```python
from build123d import *
from OCP.BRepFilletAPI import BRepFilletAPI_MakeChamfer

# Parameters (mm, degrees)
BOSS_EXTRUDE1_DEPTH = 3
CHAMFER1_SIZE       = 3
CHAMFER1_SIZE_2     = 1.853922924
SKETCH7_R           = 2
CUT_EXTRUDE6_DEPTH  = 1.5
SKETCH9_R           = 2
CUT_EXTRUDE7_DEPTH  = 1.5
SKETCH12_R          = 2
CUT_EXTRUDE8_DEPTH  = 1.5
SKETCH11_R          = 2
CUT_EXTRUDE9_DEPTH  = 1.5
SKETCH10_R          = 2
CUT_EXTRUDE10_DEPTH = 1.5


with BuildPart() as part:
    # Sketch1 → Boss-Extrude1 (new body)
    with BuildSketch(Plane(origin=(0, 0, 0), x_dir=(1, 0, 0), z_dir=(0, 1, 0))):
        Polygon((61.803398875, 0), (19.098300563, 58.778525229), (-50, 36.3271264), (-50, -36.3271264), (19.098300563, -58.778525229), align=None)
    extrude(amount=BOSS_EXTRUDE1_DEPTH)

    # Chamfer1
    chamfer1_edges_1 = [part.edges().sort_by_distance(p)[0] for p in [
        (-50, 3, 0),
    ]]
    chamfer1_side_1 = [part.faces().sort_by_distance(p)[0] for p in [
        (-50, 2.962921542, 0),
    ]]
    chamfer1_edges_2 = [part.edges().sort_by_distance(p)[0] for p in [
        (-15.450849719, 3, -47.552825815),
    ]]
    chamfer1_side_2 = [part.faces().sort_by_distance(p)[0] for p in [
        (-15.450849719, 2.962921542, -47.552825815),
    ]]
    chamfer1_edges_3 = [part.edges().sort_by_distance(p)[0] for p in [
        (40.450849719, 3, -29.389262615),
    ]]
    chamfer1_side_3 = [part.faces().sort_by_distance(p)[0] for p in [
        (40.450849719, 2.962921542, -29.389262615),
    ]]
    chamfer1_edges_4 = [part.edges().sort_by_distance(p)[0] for p in [
        (40.450849719, 3, 29.389262615),
    ]]
    chamfer1_side_4 = [part.faces().sort_by_distance(p)[0] for p in [
        (40.450849719, 2.962921542, 29.389262615),
    ]]
    chamfer1_edges_5 = [part.edges().sort_by_distance(p)[0] for p in [
        (-15.450849719, 3, 47.552825815),
    ]]
    chamfer1_side_5 = [part.faces().sort_by_distance(p)[0] for p in [
        (-15.450849719, 2.962921542, 47.552825815),
    ]]
    chamfer1 = BRepFilletAPI_MakeChamfer(part.part.solid().wrapped)
    for e in chamfer1_edges_1:
        chamfer1.Add(CHAMFER1_SIZE - 0.0001, CHAMFER1_SIZE_2 - 0.0001, e.wrapped, chamfer1_side_1[0].wrapped)
    for e in chamfer1_edges_2:
        chamfer1.Add(CHAMFER1_SIZE - 0.0001, CHAMFER1_SIZE_2 - 0.0001, e.wrapped, chamfer1_side_2[0].wrapped)
    for e in chamfer1_edges_3:
        chamfer1.Add(CHAMFER1_SIZE - 0.0001, CHAMFER1_SIZE_2 - 0.0001, e.wrapped, chamfer1_side_3[0].wrapped)
    for e in chamfer1_edges_4:
        chamfer1.Add(CHAMFER1_SIZE - 0.0001, CHAMFER1_SIZE_2 - 0.0001, e.wrapped, chamfer1_side_4[0].wrapped)
    for e in chamfer1_edges_5:
        chamfer1.Add(CHAMFER1_SIZE - 0.0001, CHAMFER1_SIZE_2 - 0.0001, e.wrapped, chamfer1_side_5[0].wrapped)
    add(Compound.cast(chamfer1.Shape()), mode=Mode.REPLACE)  # a hair under: the kernel refuses the full size

    # Sketch7 → Cut-Extrude6 (cut, along a direction that is not the sketch's normal)
    with BuildSketch(Plane.XZ):
        with Locations((16.806504495, -51.725102202)):
            Circle(SKETCH7_R)
    extrude(amount=-CUT_EXTRUDE6_DEPTH, dir=(0.18758103429764753, -0.7946827516361076, -0.5773150611441635), mode=Mode.SUBTRACT)

    # Sketch9 → Cut-Extrude7 (cut, along a direction that is not the sketch's normal)
    with BuildSketch(Plane.XZ):
        with Locations((-44, -31.967871232)):
            Circle(SKETCH9_R)
    extrude(amount=-CUT_EXTRUDE7_DEPTH, dir=(-0.4910935234360889, -0.7946827516361092, -0.356800330004317), mode=Mode.SUBTRACT)

    # Sketch12 → Cut-Extrude8 (cut, along a direction that is not the sketch's normal)
    with BuildSketch(Plane.XZ):
        with Locations((-44, 31.967871232)):
            Circle(SKETCH12_R)
    extrude(amount=-CUT_EXTRUDE8_DEPTH, dir=(-0.4910935234360893, -0.7946827516361098, 0.35680033000431516), mode=Mode.SUBTRACT)

    # Sketch11 → Cut-Extrude9 (cut, along a direction that is not the sketch's normal)
    with BuildSketch(Plane.XZ):
        with Locations((16.806504495, 51.725102202)):
            Circle(SKETCH11_R)
    extrude(amount=-CUT_EXTRUDE9_DEPTH, dir=(0.18758103429764547, -0.7946827516361094, 0.577315061144162), mode=Mode.SUBTRACT)

    # Sketch10 → Cut-Extrude10 (cut, along a direction that is not the sketch's normal)
    with BuildSketch(Plane.XZ):
        with Locations((54.38699101, 0)):
            Circle(SKETCH10_R)
    extrude(amount=-CUT_EXTRUDE10_DEPTH, dir=(0.607024978276895, -0.7946827516361074, -2.948455894095108e-15), mode=Mode.SUBTRACT)


solid = part.part
```
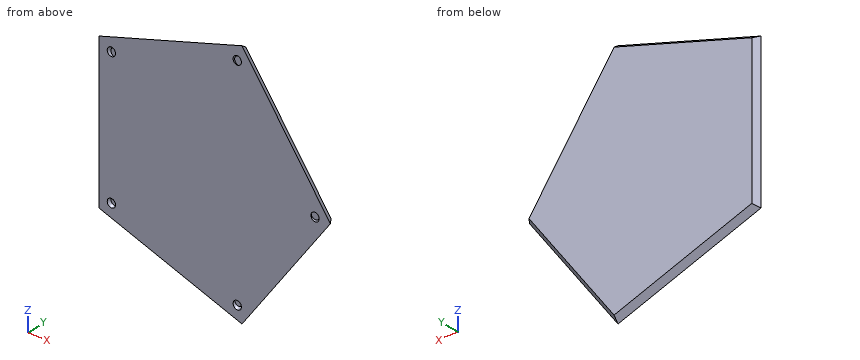
Here's how the part is built. I have some questions about the finished solid (model axes, mm). Coordinates: 2 decimals unless noted, no trailing zeros. Order: outer loops, then holes, each group sorted by start corner. A loop starts at its lowest first (then second) coordinate and runs counter-clockwise, first axis right, second up.
1) Will these pins go through, and if not, where does the flat tip stop? pin 1 (1.2 mm diameter, centred on x = 17, z = 50, fed in from -Y); pin 2 (1 mm diameter, centred on x = 2, y = 0.5, fed in from -Z); pin 3 (1.2 mm diameter, centred on x = -44, z = -32, fed in from -Y); pin 4 (1 mm diameter, centred on y = 1.5, z = -13, fed in from -X).
2) I need wall thicknesses on line 1 (Z direction, x = -43.5, y = 0.95); line 2 (Z direction, x = 40, y = 1.25); line 3 (Z direction, x = 42.5, y = 2.25). Which ranges of each line are inside material? Lowest first, please.
3) Imagine slicing it at A-A on y = 1.75. List the corners of the cut face in (x, z) for me, and give its area (3 significant figures).
Response values:
1. pin 1: stops at y = 0
1. pin 2: stops at z = -53.26
1. pin 3: stops at y = 1.19
1. pin 4: stops at x = -49.38
2. line 1: z = -37.82 to -33.54, -29.54 to 29.54, 33.54 to 37.82
2. line 2: z = -28.7 to 28.7
2. line 3: z = -24.2 to 24.2
3. outline: (-48.92, -35.54) - (18.69, -57.51) - (60.47, 0) - (18.69, 57.51) - (-48.92, 35.54) - close
3. area: 8,690 mm2
